```python
from build123d import *

# Parameters (mm, degrees)
BOSS_EXTRUDE1_DEPTH = 20


with BuildPart() as part:
    # Sketch2 → Boss-Extrude1 (new body)
    with BuildSketch(Plane(origin=(0, 0, 0), x_dir=(1, 0, 0), z_dir=(0, 1, 0))):
        with BuildLine():
            ThreePointArc((6, 0), (0, -6), (-6, 0))
            Line((-6, 0), (-6, 26.837473801))
            ThreePointArc((-6, 26.837473801), (-17.193748864, -21.462176031), (27.5, 0))
            ThreePointArc((27.5, 0), (21.462176031, 17.193748864), (6, 26.837473801))
            Line((6, 26.837473801), (6, 0))
        make_face()
    extrude(amount=BOSS_EXTRUDE1_DEPTH)


solid = part.part
```
For this review, take the finished solid that the model builds, in its own axes (mm). A direction names the side the tool comes from. Give positions to 0.01 mm unless a question says otherwise; leave off trailing zeros. Order: outer loops, then holes, each group sorted by start corner. A loop starts at its lowest first (then second) coordinate and runs counter-clockwise, first axis right, second up.
1) Take a section at A-A (z = -19). Give the boundary of the cut face in (x, y), then the cut area to 3 significant figures.
2) Take a section at B-B (y = 5.75). Give the boundary of the cut face in (x, z).
3) Take a section at C-C (x = 0). Give the boundary of the cut face in (y, z).
4) Take a section at D-D (z = 4). Give the boundary of the cut face in (x, y), then the cut area to 3 significant figures.
5) The part is to be moulded in two halves that separate along X. For faces 1 (the face through (-6, 10, -13)), 2 (the face through (-6.5, 20, 0)), say which applies: released by +X, released by -X, zero draft, split by the parting line, or undercut.
6) For faces 3 (the face through (6, 10, -14)), 4 (the face through (-6.5, 0, 0)), list the 3-axis set-ups (+Z, -Z, +X, -X, +Y, -Y) from which the entire face can be reached by the end or side of a thin tool; tool diameter is ignored.
7) Wall thickness on line 1 (X direction, y = 7.25, z = -20); line 2 (X direction, y = 3, z = -19); line 3 (Z direction, x = 0, y = 2.5): over which ranges is each line inside the solid? List them lowest first.
8) Insertion check: pin 1 (1.5 mm diameter, centred on x = 14.5, y = 12.5, fed in from -Z); pin 2 (8 mm diameter, centred on x = -19, z = -18, fed in from -Y); pin 3 (10 mm diameter, centred on x = -19.5, y = 4, fed in from +Z); pin 4 (1.5 mm diameter, centred on x = -3.5, y = 13.5, fed in from -Z). Each pin has a flat end and moves straight along its axis. Give the tip position at first contact, or say it passes through.
Derived:
1. outline: (-19.88, 0) - (-6, 0) - (-6, 20) - (-19.88, 20) - close; (6, 0) - (19.88, 0) - (19.88, 20) - (6, 20) - close
1. area: 555 mm2
2. outline: (-6, -26.84) - (-6, 0) arc R6 cw to (6, 0) - (6, -26.84) arc R27.5 ccw (long way) to start
3. outline: (0, 6) - (20, 6) - (20, 27.5) - (0, 27.5) - close
4. outline: (-27.21, 0) - (-4.47, 0) - (-4.47, 20) - (-27.21, 20) - close; (4.47, 0) - (27.21, 0) - (27.21, 20) - (4.47, 20) - close
4. area: 909 mm2
5. face 1: undercut
5. face 2: zero draft
6. face 3: -Z, +Y, -Y
6. face 4: +Z, -Z, +X, -X, -Y
7. line 1: x = -18.87 to -6, 6 to 18.87
7. line 2: x = -19.88 to -6, 6 to 19.88
7. line 3: z = 6 to 27.5
8. pin 1: stops at z = -23.82
8. pin 2: stops at y = 0
8. pin 3: stops at z = 23.37
8. pin 4: stops at z = 4.24
